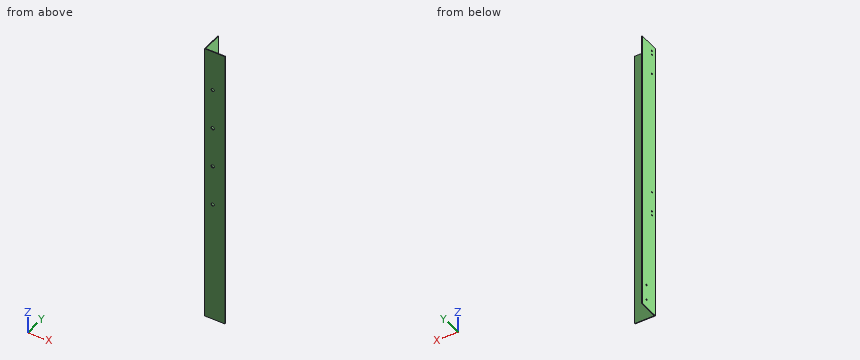
from build123d import *

# Parameters (mm, degrees)
EXTRUDE_1_DEPTH             = 700
SKETCH_2_R                  = 4
CUT_EXTRUDE_1_DEPTH         = 10
SKETCH_3_R                  = 2.25
CUT_EXTRUDE_2_DEPTH         = 51
HOLE_WIZARD_3_5_3_5_1_D     = 3.5
HOLE_WIZARD_3_5_3_5_1_DEPTH = 2
HOLE_WIZARD_3_5_3_5_1_TIP   = 1.051506083


with BuildPart() as part:
    # 草圖1 → 填料-伸長1 (new body)
    with BuildSketch(Plane.XY):
        Polygon((0, 50), (0, 0), (50, 0), (50, 1.8), (1.8, 1.8), (1.8, 50), align=None)
    extrude(amount=EXTRUDE_1_DEPTH)

    # 草圖2 → 除料-伸長1 (cut)
    with BuildSketch(Plane(origin=(0, 0, 0), x_dir=(-1, 0, 0), z_dir=(0, -1, 0))):
        with Locations((-20, -300)):
            Circle(SKETCH_2_R)
        with Locations((-20, -600)):
            Circle(SKETCH_2_R)
        with Locations((-20, -500)):
            Circle(SKETCH_2_R)
        with Locations((-20, -400)):
            Circle(SKETCH_2_R)
    extrude(amount=-CUT_EXTRUDE_1_DEPTH, mode=Mode.SUBTRACT)

    # 草圖3 → 除料-伸長2 (cut, through all)
    with BuildSketch(Plane.ZY):
        with Locations((58.34, 33.5)):
            Circle(SKETCH_3_R)
        with Locations((20, 33.5)):
            Circle(SKETCH_3_R)
    extrude(amount=-CUT_EXTRUDE_2_DEPTH, mode=Mode.SUBTRACT)

    # Ø3.5 (3.5) 直徑孔1
    with Locations(Plane.ZY):
        with Locations((685, 13.5), (675, 13.5), (625, 13.5), (255, 13.5), (265, 13.5), (315, 13.5)):
            Hole(HOLE_WIZARD_3_5_3_5_1_D / 2, depth=HOLE_WIZARD_3_5_3_5_1_DEPTH)
            with Locations((0, 0, -(HOLE_WIZARD_3_5_3_5_1_DEPTH + HOLE_WIZARD_3_5_3_5_1_TIP / 2))):  # 118° drill point
                Cone(0, HOLE_WIZARD_3_5_3_5_1_D / 2, HOLE_WIZARD_3_5_3_5_1_TIP, mode=Mode.SUBTRACT)


solid = part.part
Source: CAD feature listing. Evaluate the final solid. Frame: model axes, mm. Give positions to 0.01 mm unless a question says otherwise; leave off trailing zeros. Order: outer loops, then holes, each group sorted by start corner. A loop starts at its lowest first (then second) coordinate and runs counter-clockwise, first axis right, second up. Notation, with made-up numbers: (-35, -8.5) -> (1, -8.5) arc R31 cw to (1, 18.5) -> close; hole circle Ø9 at (-39, 45). An arc over 180 degrees is marked (long way). Use a Markdown table: item, result.
1) Contact query for flat-ended pins moving along their axis: P1, Ø24, axis at y = 33, z = 350, coming from the +X side; P2, Ø14.5, axis at x = 31.5, z = 271, coming from the +Y side. Output: stop coordinate, or through.
Answer list:
| item | result |
|---|---|
| P1 | x = 1.8 |
| P2 | y = 1.8 |
2) Ray query, line 1 along X through (y, z) = (1, 300); line 2 along Y through (x, z) = (1.2, 315); line 3 along Y through (x, z) = (1.3, 58.34). Return the intervals inside material, ascending. Write a range as [from, to].
Answer list:
| item | result |
|---|---|
| line 1 | [0, 16], [24, 50] |
| line 2 | [0, 11.75], [15.25, 50] |
| line 3 | [0, 31.25], [35.75, 50] |
3) Section query A-A, the plane z = 175. Return the cut outline in (x, y), then the cut area to 3 significant figures.
Answer list:
| item | result |
|---|---|
| outline | (0, 0) -> (50, 0) -> (50, 1.8) -> (1.8, 1.8) -> (1.8, 50) -> (0, 50) -> close |
| area | 177 mm² |
